Autodesk Inventor part; units mm, degrees
ref_plane "YZ Plane" through (0, 0, 0) normal (1, 0, 0) x (0, 1, 0)
ref_plane "XZ Plane" through (0, 0, 0) normal (0, 1, 0) x (-1, 0, 0)
ref_plane "XY Plane" through (0, 0, 0) normal (0, 0, 1) x (1, 0, 0)
sketch "Sketch1" plane through (0, 0, 0) normal (0, 0, 1) x (1, 0, 0)
  line L0 (-15, -0.0024) -> (15, -0.0024)
  line L1 (15, -0.0024) -> (15, 4.9976)
  line L2 (15, 4.9976) -> (-15, 4.9976)
  line L3 (-15, 4.9976) -> (-15, -0.0024)
  line L4 (-7.5, -0.0024) -> (7.5, -0.0024)
  line L5 (7.5, -0.0024) -> (7.5, -142.5024)
  line L6 (7.5, -142.5024) -> (-7.5, -142.5024)
  line L7 (-7.5, -142.5024) -> (-7.5, -0.0024)
  point P0 (0, 0)
  point P1 (0, -0.0024)
  point P2 (7.5, -0.0024)
  dimension "d0" = 5
  dimension "d1" = 147.5
  dimension "d3" = 7.5
  dimension "d5" = 30
  dimension "d6" = 15
  dimension "d7" = 7.5
extrude "Extrusion1" add sketch "Sketch1" along normal blind 10
sketch "Sketch2" plane through (0, 0, 10) normal (0, 0, 1) x (1, 0, 0)
  line L0 (-3.5, 0) -> (3.5, 0)
  line L1 (3.5, 0) -> (3.5, -137.5024)
  line L2 (3.5, -137.5024) -> (-3.5, -137.5024)
  line L3 (-3.5, -137.5024) -> (-3.5, 0)
  line L4 (-7.5, -0.0024) -> (-7.5, -142.5024)
  line L5 (7.5, -142.5024) -> (7.5, -0.0024)
  line L6 (-7.5, -142.5024) -> (7.5, -142.5024)
  line L7 (-3.5, -68.7512) -> (3.5, -68.7512)
  line L8 (3.5, -68.7512) -> (3.5, -73.7512)
  line L9 (3.5, -73.7512) -> (-3.5, -73.7512)
  line L10 (-3.5, -73.7512) -> (-3.5, -68.7512)
  point P0 (0, 0)
  point P1 (3.5, -68.7512)
  dimension "d10" = 4
  dimension "d11" = 4
  dimension "d12" = 5
  dimension "d13" = 5
extrude "Extrusion2" cut sketch "Sketch2" against normal blind 10 contours L0 L1 L7 L3 | L9 L1 L2 L3
sketch "Sketch3" plane through (7.5, -0.0024, 0) normal (0, -1, 0) x (1, 0, 0)
  circle A0 centre (4, 5) radius 1.5
  circle A1 centre (-19, 5) radius 1.5
  line L0 (7.5, 0) -> (7.5, 10)
  line L1 (0, 10) -> (7.5, 10)
  line L2 (-22.5, 10) -> (-15, 10)
  line L3 (-22.5, 0) -> (-22.5, 10)
  point P0 (-7.5, 0)
  point P1 (-18.75, 10)
  dimension "d16" = 3.5
  dimension "d17" = 5
  dimension "d19" = 5
  dimension "d20" = 3.5
  dimension "d21" = 3
  dimension "d22" = 3
extrude "Extrusion3" cut sketch "Sketch3" against normal blind 10
chamfer "Chamfer1" distance 1.5 angle 45 2 edges at (-13, -0.0024, 5) (10, -0.0024, 5)
properties part number "CenterSupport"
Here's how the part is built. I have some questions about the finished solid (model axes, mm). A direction names the side the tool comes from. Round coordinates to 2 decimals unless told otherwise and drop trailing zeros. Order: outer loops, then holes, each group sorted by start corner. A loop starts at its lowest first (then second) coordinate and runs counter-clockwise, first axis right, second up. Notation, with made-up numbers: M -30.5,-17 L 5.5,-17 A37 ccw 5.5,21 Z; hole C 30,2.5 d2. An arc over 180 degrees is marked long. Return JSON: item names as keys, results as strings. Group by question number.
1. If we section it at B-B on y = -21: List the corners of the cut face in (x, z) for me.
2. On a 3-axis mill with a long thin cutter (end or side, diameter ignored), from which of +Z, -Z, +X, -X, +Y, -Y can I reach the whole of each face in a straight line? I mean faces 5 (the face through (10, 3, 5)), 6 (the face through (0, -68.751, 5)). Say none if no direction works.
3. If we section it at C-C on z = 5: List the corners of the cut face in (x, y) for me.
4. Please list where these lines run through material, in increasing order: probe 1 along Y at (x, z) = (1, 7.25); probe 2 along X at (y, z) = (-127.5, 8.5); probe 3 along Z at (x, y) = (-11.5, 3.1).
5. If we section it at D-D on x = 11.5: List the corners of the cut face in (y, z) for me, then the cut area to 4 significant figures.
6. I'm going to push flat-ended pins straight in: pin 1 Ø1 at (y, z) = (-105, 5.5) entering from +X; pin 2 Ø6 at (y, z) = (-22, 3.5) entering from -X; pin 3 Ø2 at (x, z) = (-11.5, 2.5) entering from -Y. Where does each tip first touch, or does it pass through?
7. If we section it at A-A on x = 0: List the corners of the cut face in (y, z) for me.
8. If we mould it in two halves opening along Y, with no side actions, what happens to faces 1 (the face through (15, 2, 5)), 2 (the face through (0, 4.998, 5)), 3 (the face through (-11.3, -0.002, 1.6)), 4 (the face through (-3.5, -35, 5))? For each: pulls with the +Y half, pulls with the -Y half, needs draft (parallel to the pull), parting line crosses it, or undercut.
Reply:
{
 "1": {"outline": "M -7.5,0 L -3.5,0 L -3.5,10 L -7.5,10 Z; M 3.5,0 L 7.5,0 L 7.5,10 L 3.5,10 Z"},
 "2": {"face 5": "+Y, -Y", "face 6": "+Z, -Z"},
 "3": {"outline": "M -15,0 L -14.5,0 L -13,1.5 L -13,5 L -15,5 Z; M -10,1.5 L -8.5,0 L -7.5,0 L -7.5,-142.5 L 7.5,-142.5 L 7.5,0 L 8.5,0 L 10,1.5 L 10,5 L -10,5 Z; M 13,1.5 L 14.5,0 L 15,0 L 15,5 L 13,5 Z; hole M -3.5,-137.5 L 3.5,-137.5 L 3.5,-73.75 L -3.5,-73.75 Z; hole M -3.5,-68.75 L 3.5,-68.75 L 3.5,0 L -3.5,0 Z"},
 "4": {"probe 1": "-142.5 to -137.5, -73.75 to -68.75, 0 to 5", "probe 2": "-7.5 to -3.5, 3.5 to 7.5", "probe 3": "0 to 3.5, 6.5 to 10"},
 "5": {"outline": "M 0,0 L 5,0 L 5,3.5 L 1.5,3.5 L 0,2 Z; M 0,8 L 1.5,6.5 L 5,6.5 L 5,10 L 0,10 Z", "area": "32.75 mm^2"},
 "6": {"pin 1": "x = 7.5", "pin 2": "x = -7.5", "pin 3": "y = 0"},
 "7": {"outline": "M -142.5,0 L -137.5,0 L -137.5,10 L -142.5,10 Z; M -73.75,0 L -68.75,0 L -68.75,10 L -73.75,10 Z; M 0,0 L 5,0 L 5,10 L 0,10 Z"},
 "8": {"face 1": "needs draft", "face 2": "pulls with the +Y half", "face 3": "pulls with the -Y half", "face 4": "undercut"}
}
